Read the model definition and answer for the solid it produces. Units are mm, in the model's axes. A direction names the side the tool comes from. Give positions to 0.01 mm unless a question says otherwise; leave off trailing zeros. Write each loop counter-clockwise with the first axis right and the second up, starting at its lowest first coordinate (ties: lowest second). Pieces come first, ordered by that corner, then holes.
Solid Edge part; units mm, degrees
sketch "Sketch1" plane through (0, 0, 0) normal (0, -1, 0) x (1, 0, 0)
  line L0 (13.4324, 3.2075) -> (-1.253, 3.2075)
  line L1 (-1.253, 3.2075) -> (-0.0083, 2.3972)
  arc A0 (-0.0083, 2.3972) -> (0.7346, 2.1301) centre (0.9285, 3.8363) ccw
  line L2 (0.7346, 2.1301) -> (2.1383, 1.9706)
  arc A1 (2.1383, 1.9706) -> (0.8387, -1.6081) centre (1.5999, 0.1408) cw
  line L3 (-1.3928, -0.6369) -> (0.8387, -1.6081)
  arc A2 (-5.4369, 2.7406) -> (-1.3928, -0.6369) centre (2.3423, 7.9454) ccw
  line L4 (-5.7493, 3.2075) -> (-5.4369, 2.7406)
  line L5 (-5.7493, 3.2075) -> (-10.2791, 3.2075)
  line L6 (-10.2791, 3.2075) -> (-10.2791, -3.2075)
  line L7 (-10.2791, -3.2075) -> (13.4324, -3.2075)
  line L8 (13.4324, -3.2075) -> (13.4324, 3.2075)
extrude "Protrusion1" add sketch "Sketch1" against normal blind 24
sketch "Sketch2" plane through (4.513, 12, 3.2075) normal (0, 0, 1) x (1, 0, 0)
  line L0 (-14.7921, 7.5) -> (3.4988, 7.5)
  line L1 (3.4988, 7.5) -> (3.4988, -7.5)
  line L2 (-14.7921, -7.5) -> (3.4988, -7.5)
  line L3 (-14.7921, 7.5) -> (-14.7921, -7.5)
extrude "Cutout1" cut sketch "Sketch2" against normal blind 4.4
sketch "Sketch3" plane through (1.5766, 0, 0) normal (0, -1, 0) x (1, 0, 0)
  circle A0 centre (0.0232, 0.1408) radius 1.9073
extrude "ScavoEstrusione_2" cut sketch "Sketch3" against normal blind 40.5632
Item 1: Section B-B (y = 14.75) is taken. Write down the section's boundary in (x, z).
Result set:
outline: (-10.28, -3.21) - (13.43, -3.21) - (13.43, 3.21) - (8.01, 3.21) - (8.01, -1.19) - (2.96, -1.19) arc R1.91 cw to (0.84, -1.61) - (-0.12, -1.19) - (-10.28, -1.19) - close
Item 2: Which of the six approach directions +Z, -Z, +X, -X, +Y, -Y give full straight-line access (tool end or side, diameter ignored) to faces 5 (the flat face through (-8, 2, 3.208)), 6 (the cylindrical face through (-3.69, 2.22, 0.79)), 7 (the flat face through (4, 19.5, 2))?
Result set:
face 5: +Z, +X, -X, +Y, -Y
face 6: +Z, +Y, -Y
face 7: +Z, -X
Item 3: Section A-A (x = 5.25) is taken. Write down the section's boundary in (y, z).
Result set:
outline: (0, -3.21) - (24, -3.21) - (24, 3.21) - (19.5, 3.21) - (19.5, -1.19) - (4.5, -1.19) - (4.5, 3.21) - (0, 3.21) - close
Item 4: Find the intervals of material crossed by line 1 along Y through (x, z) = (-8, 1.75); line 2 along X through (y, z) = (10, 1.25); line 3 along Z through (x, y) = (5.75, 13.5), in increasing order.
Result set:
line 1: y = 0 to 4.5, 19.5 to 24
line 2: x = 8.01 to 13.43
line 3: z = -3.21 to -1.19
Item 5: Determine the mould class of faces 1 (the flat face through (2, 24, -2)), 2 (the flat face through (-0.64, 2.22, 2.81)), 3 (the flat face through (-0.64, 21.72, 2.81)), 4 (the cylindrical face through (-3.69, 21.72, 0.79)) for opening direction Z: pulls with the +Z half, pulls with the -Z half, needs draft (parallel to the pull), parting line crosses it, or undercut.
Result set:
face 1: needs draft
face 2: undercut
face 3: undercut
face 4: pulls with the +Z half
Item 6: Each of these flat-tipped pins is pushed along its axis until it touches: pin 1 Ø1.5 at (x, y) = (6, 13) entering from +Z; pin 2 Ø1.3 at (y, z) = (9, 1.5) entering from -X; pin 3 Ø3 at (x, z) = (1, 0.5) entering from -Y. Where does it stop, or does it pass through?
Result set:
pin 1: stops at z = -1.19
pin 2: stops at x = 8.01
pin 3: passes through
Item 7: Section C-C (z = 0.25) is taken. Write down the section's boundary in (x, y).
Result set:
outline: (-10.28, 0) - (-2.99, 0) - (-2.99, 4.5) - (-10.28, 4.5) - close; (-10.28, 19.5) - (-2.99, 19.5) - (-2.99, 24) - (-10.28, 24) - close; (3.5, 0) - (13.43, 0) - (13.43, 24) - (3.5, 24) - (3.5, 19.5) - (8.01, 19.5) - (8.01, 4.5) - (3.5, 4.5) - close
